Part model, mm, in its own coordinate system. Round coordinates to 2 decimals unless told otherwise and drop trailing zeros. Order: outer loops, then holes, each group sorted by start corner. A loop starts at its lowest first (then second) coordinate and runs counter-clockwise, first axis right, second up. Notation, with made-up numbers: (64.5, 7) -> (112.5, 7) arc R20 cw to (112.5, 22) -> close; hole circle Ø7 at (6.5, 66.5). An arc over 180 degrees is marked (long way). Return JSON: item names as keys, results as strings. Group by question number.
from build123d import *

# Parameters (mm, degrees)
SKETCH1_W           = 210
SKETCH1_H           = 88.5
SKETCH1_R           = 2.75
SKETCH1_R_2         = 2.6
BOSS_EXTRUDE1_DEPTH = 3
SKETCH2_W           = 210
SKETCH2_H           = 2.6
CUT_EXTRUDE1_DEPTH  = 1


with BuildPart() as part:
    # Sketch1 → Boss-Extrude1 (new, symmetric)
    with BuildSketch(Plane(origin=(0, 0, 0), x_dir=(1, 0, 0), z_dir=(0, 1, 0))):
        Rectangle(SKETCH1_W, SKETCH1_H)
        with Locations(Location((80, 0, 0), (0, 0, 270))):
            Circle(SKETCH1_R, mode=Mode.SUBTRACT)
        with Locations(Location((0, 0, 0), (0, 0, 270))):
            Circle(SKETCH1_R, mode=Mode.SUBTRACT)
        with Locations(Location((-80, 0, 0), (0, 0, 90))):
            Circle(SKETCH1_R, mode=Mode.SUBTRACT)
        with Locations(Location((-95, 25, 0), (0, 0, 270))):
            Circle(SKETCH1_R_2, mode=Mode.SUBTRACT)
        with Locations(Location((95, -25, 0), (0, 0, 270))):
            Circle(SKETCH1_R_2, mode=Mode.SUBTRACT)
    extrude(amount=BOSS_EXTRUDE1_DEPTH, both=True)

    # Sketch2 → Cut-Extrude1 (cut)
    with BuildSketch(Plane(origin=(0, 3, 0), x_dir=(1, 0, 0), z_dir=(0, 1, 0))):
        with Locations((0, 39.55)):
            Rectangle(SKETCH2_W, SKETCH2_H)
        with Locations((0, -39.55)):
            Rectangle(SKETCH2_W, SKETCH2_H)
    cut_extrude1 = extrude(amount=-CUT_EXTRUDE1_DEPTH, mode=Mode.SUBTRACT)

    # Mirror1: Cut-Extrude1 across plane
    add(cut_extrude1.mirror(Plane.ZX), mode=Mode.SUBTRACT)


solid = part.part
(1) Pin check, flat tips, straight feed: P1, Ø3.5, axis at x = 80, z = 0, coming from the +Y side; P2, Ø3, axis at x = 27, z = 40, coming from the +Y side; P3, Ø0.8, axis at x = 12.5, z = 39.5, coming from the -Y side; P4, Ø0.8, axis at x = -3.5, z = -40, coming from the +Y side. Stop position of each tip, or through.
(2) Saw through at A-A, the plane z = 25. List the corners of the cut face in (x, y).
(3) Mould opens along X. For faces 1 (the flat face through (-1, 0, -44.25)), 2 (the cylindrical face through (77.315, -0.042, -0.596)), 3 (the flat face through (-105, 0, 1)) say: pulls with the +X half, pulls with the -X half, needs draft (parallel to the pull), parting line crosses it, or undercut.
(4) Saw through at C-C, the plane z = 0. List the corners of the cut face in (x, y).
(5) Saw through at D-D, the plane x = 25.5. List the corners of the cut face in (y, z), and give its area (3 significant figures).
(6) Probe L1, parallel to X at y = -1.2, z = 25; L2, parallel to X at y = 0.5, z = 0; L3, parallel to Z at x = -80, y = -1.25. List the from-to ranges inside material, lowest first. Write a range as [from, to].
(7) Saw through at B-B, the plane x = -80. List the corners of the cut face in (y, z).
Results are:
{
 "1": {"P1": "passes through", "P2": "stops at y = 3", "P3": "stops at y = -2", "P4": "stops at y = 2"},
 "2": {"outline": "(-105, -3) -> (92.4, -3) -> (92.4, 3) -> (-105, 3) -> close; (97.6, -3) -> (105, -3) -> (105, 3) -> (97.6, 3) -> close"},
 "3": {"face 1": "needs draft", "face 2": "undercut", "face 3": "pulls with the -X half"},
 "4": {"outline": "(-105, -3) -> (-82.75, -3) -> (-82.75, 3) -> (-105, 3) -> close; (-77.25, -3) -> (-2.75, -3) -> (-2.75, 3) -> (-77.25, 3) -> close; (2.75, -3) -> (77.25, -3) -> (77.25, 3) -> (2.75, 3) -> close; (82.75, -3) -> (105, -3) -> (105, 3) -> (82.75, 3) -> close"},
 "5": {"outline": "(-3, -44.25) -> (3, -44.25) -> (3, -40.85) -> (2, -40.85) -> (2, -38.25) -> (3, -38.25) -> (3, 38.25) -> (2, 38.25) -> (2, 40.85) -> (3, 40.85) -> (3, 44.25) -> (-3, 44.25) -> (-3, 40.85) -> (-2, 40.85) -> (-2, 38.25) -> (-3, 38.25) -> (-3, -38.25) -> (-2, -38.25) -> (-2, -40.85) -> (-3, -40.85) -> close", "area": "521 mm^2"},
 "6": {"L1": "x = [-105, 92.4], [97.6, 105]", "L2": "x = [-105, -82.75], [-77.25, -2.75], [2.75, 77.25], [82.75, 105]", "L3": "z = [-44.25, -2.75], [2.75, 44.25]"},
 "7": {"outline": "(-3, -44.25) -> (3, -44.25) -> (3, -40.85) -> (2, -40.85) -> (2, -38.25) -> (3, -38.25) -> (3, -2.75) -> (-3, -2.75) -> (-3, -38.25) -> (-2, -38.25) -> (-2, -40.85) -> (-3, -40.85) -> close; (-3, 2.75) -> (3, 2.75) -> (3, 38.25) -> (2, 38.25) -> (2, 40.85) -> (3, 40.85) -> (3, 44.25) -> (-3, 44.25) -> (-3, 40.85) -> (-2, 40.85) -> (-2, 38.25) -> (-3, 38.25) -> close"}
}
